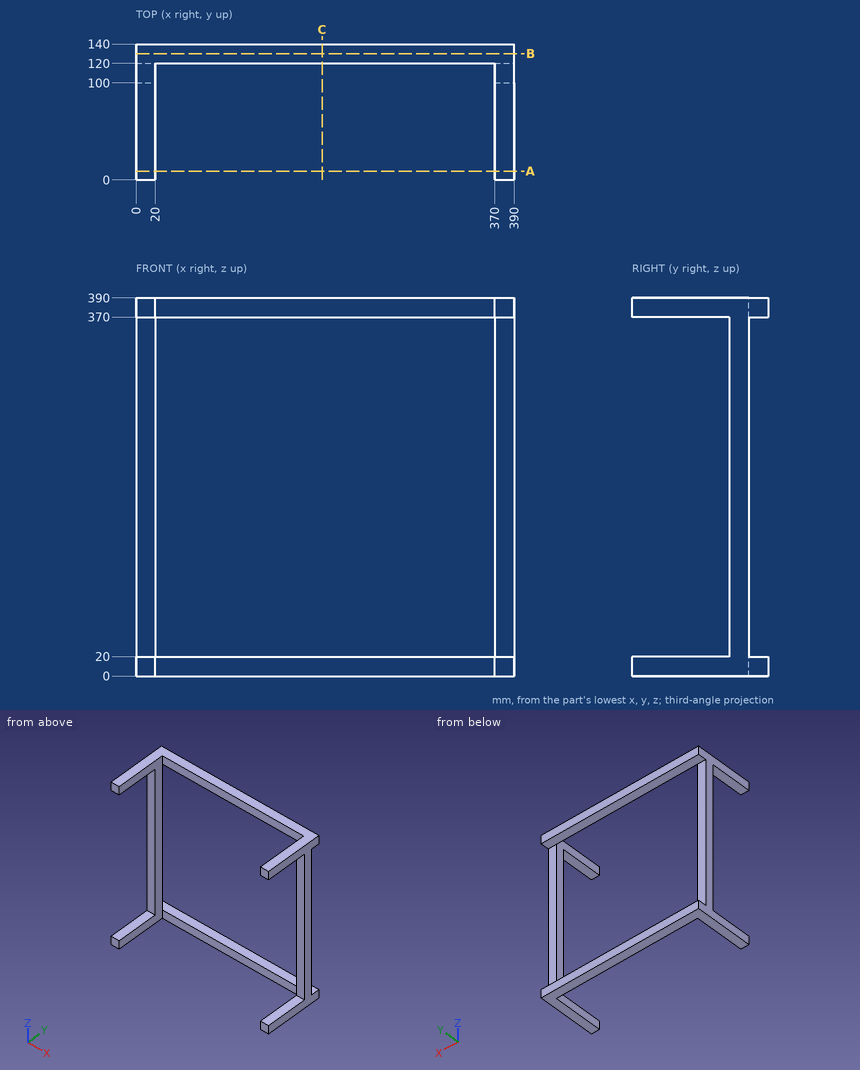
Can you work these out from the drawing? Everything is in mm from the part's minimum corner. Round coordinates to 2 decimals unless told otherwise and drop trailing zeros. Loops run counter-clockwise (first coordinate to the right, second up) from the corner with the lowest first, then second, coordinate; pieces in that order, holes last. Notation, with made-up numbers: (-38.75, -30) -> (-28.75, -30) arc R16 ccw to (-28.75, -8) -> close; hole circle Ø11 at (87.5, -13.75). An arc over 180 degrees is marked (long way). Answer in a Markdown table with one row per item.
Item 1: Will these pins go through, and if not, where does the flat tip stop? P1, Ø10, axis at x = 14.5, z = 230.5, coming from the +Y side; P2, Ø16, axis at x = 173.5, z = 5, coming from the -Y side; P3, Ø6, axis at x = 382.5, z = 189.5, coming from the -Y side; P4, Ø16, axis at x = 7, y = 33.5, coming from the -Z side.
Answer block:
| item | result |
|---|---|
| P1 | y = 120 |
| P2 | y = 120 |
| P3 | y = 100 |
| P4 | z = 0 |
Item 2: Suppose I cut it at C-C, the plane x = 192. List the corners of the cut face in (y, z) for me, plus the area to 3 significant figures.
Answer block:
| item | result |
|---|---|
| outline | (120, 0) -> (140, 0) -> (140, 20) -> (120, 20) -> close; (120, 370) -> (140, 370) -> (140, 390) -> (120, 390) -> close |
| area | 800 mm² |
Item 3: If I drill on probe 1 along X at (y, z) = (117.5, 217.5), over which ranges is the centre line in solid material (lowest first)?
Answer block:
| item | result |
|---|---|
| probe 1 | 0 to 20, 370 to 390 |
Item 4: Suppose I cut it at A-A, the plane y = 9. List the corners of the cut face in (x, z) for me, plus the area to 3 significant figures.
Answer block:
| item | result |
|---|---|
| outline | (0, 0) -> (20, 0) -> (20, 20) -> (0, 20) -> close; (0, 370) -> (20, 370) -> (20, 390) -> (0, 390) -> close; (370, 0) -> (390, 0) -> (390, 20) -> (370, 20) -> close; (370, 370) -> (390, 370) -> (390, 390) -> (370, 390) -> close |
| area | 1,600 mm² |
Item 5: Suppose I cut it at B-B, the plane y = 130. List the corners of the cut face in (x, z) for me.
Answer block:
| item | result |
|---|---|
| outline | (0, 0) -> (390, 0) -> (390, 20) -> (0, 20) -> close; (0, 370) -> (390, 370) -> (390, 390) -> (0, 390) -> close |
